Geometry check sheet. Reference: drawing and pictorial views, mm from the part's lowest x, y, z. Round coordinates to 2 decimals unless told otherwise and drop trailing zeros. Write each loop counter-clockwise with the first axis right and the second up, starting at its lowest first coordinate (ties: lowest second). Pieces come first, ordered by that corner, then holes. Notation, with made-up numbers: M -24,34 L 3,34 A6 ccw 3,39 Z; hole C 62,5 d11. An arc over 180 degrees is marked long. Answer in a Markdown table with one row per item.
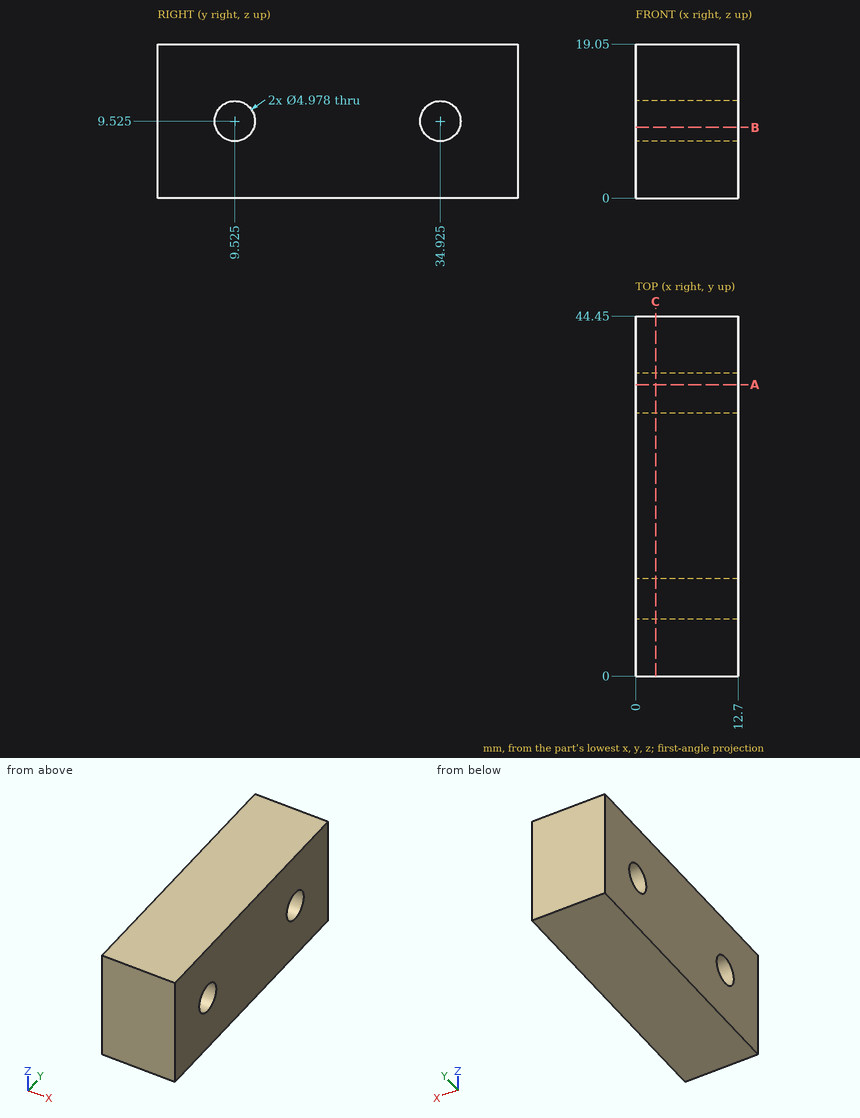
1. Section check C-C, the plane x = 2.5. Count the separate pieces of the cut face and the enclosed holes in it, and give its area (3 significant figures).
Found:
| item | result |
|---|---|
| separate pieces | 1 |
| enclosed holes | 2 |
| area | 808 mm2 |
2. Section check A-A, the plane y = 36. Record the cut outline in (x, z), and give its area (3 significant figures).
Found:
| item | result |
|---|---|
| outline | M 0,0 L 12.7,0 L 12.7,7.28 L 0,7.28 Z; M 0,11.77 L 12.7,11.77 L 12.7,19.05 L 0,19.05 Z |
| area | 185 mm2 |
3. Scan lines: L1, parallel to Y at x = 10.25, z = 7.75; L2, parallel to Y at x = 12, z = 9; L3, parallel to Z at x = 3, y = 11.5. Record each from-to range of solid material in increasing order.
Found:
| item | result |
|---|---|
| L1 | y = 0 to 7.78, 11.27 to 33.18, 36.67 to 44.45 |
| L2 | y = 0 to 7.09, 11.96 to 32.49, 37.36 to 44.45 |
| L3 | z = 0 to 8.01, 11.04 to 19.05 |
4. Section check B-B, the plane z = 8.75. Record the cut outline in (x, y).
Found:
| item | result |
|---|---|
| outline | M 0,0 L 12.7,0 L 12.7,7.16 L 0,7.16 Z; M 0,11.89 L 12.7,11.89 L 12.7,32.56 L 0,32.56 Z; M 0,37.29 L 12.7,37.29 L 12.7,44.45 L 0,44.45 Z |
